```python
from build123d import *

# Parameters (mm, degrees)
F0_R     = 1
F1_DEPTH = 36
F0_R_2   = 2
F2_DEPTH = 6
F3_R     = 1
F4_R     = 1
F5_DEPTH = 25
F7_DEPTH = 100
F8_R     = 3


with BuildPart() as f1:
    # F0 (on Top) → F1 (new body)
    with BuildSketch(Plane.XY):
        with BuildLine():
            Line((-20, -12.5), (20, -12.5))
            Line((20, -12.5), (22, -12.5))
            Line((22, -12.5), (28, -12.5))
            ThreePointArc((28, -12.5), (29.414214, -11.914214), (30, -10.5))
            Line((30, -10.5), (30, 10.5))
            ThreePointArc((30, 10.5), (29.414214, 11.914214), (28, 12.5))
            Line((28, 12.5), (22, 12.5))
            Line((22, 12.5), (20, 12.5))
            Line((20, 12.5), (-20, 12.5))
            Line((-20, 12.5), (-28, 12.5))
            ThreePointArc((-28, 12.5), (-29.414214, 11.914214), (-30, 10.5))
            Line((-30, 10.5), (-30, -10.5))
            ThreePointArc((-30, -10.5), (-29.414214, -11.914214), (-28, -12.5))
            Line((-28, -12.5), (-22, -12.5))
            Line((-22, -12.5), (-20, -12.5))
        make_face()
        with Locations((-26, -6)):
            Circle(F0_R, mode=Mode.SUBTRACT)
        with Locations((26, -6)):
            Circle(F0_R, mode=Mode.SUBTRACT)
        with Locations((-26, 6)):
            Circle(F0_R, mode=Mode.SUBTRACT)
        Polygon((20.75, -10.25), (-20.75, -10.25), (-20.75, 10.25), (20.75, 10.25), (20.75, 5), (23.25, 5), (23.25, -5), (20.75, -5), align=None, mode=Mode.SUBTRACT)
        with Locations((26, 6)):
            Circle(F0_R, mode=Mode.SUBTRACT)
    extrude(amount=F1_DEPTH)

    # F0 (on Top) → F2 (join)
    with BuildSketch(Plane.XY):
        with BuildLine():
            ThreePointArc((-22, -14.5), (-21.414214, -13.085786), (-20, -12.5))
            Line((-20, -12.5), (-22, -12.5))
            Line((-22, -12.5), (-28, -12.5))
            ThreePointArc((-28, -12.5), (-29.414214, -11.914214), (-30, -10.5))
            Line((-30, -10.5), (-30, -12.5))
            Line((-30, -12.5), (-30, -18.5))
            ThreePointArc((-30, -18.5), (-29.414214, -19.914214), (-28, -20.5))
            Line((-28, -20.5), (-24, -20.5))
            ThreePointArc((-24, -20.5), (-22.585786, -19.914214), (-22, -18.5))
            Line((-22, -18.5), (-22, -14.5))
        make_face()
        with Locations((-26, -16.5)):
            Circle(F0_R_2, mode=Mode.SUBTRACT)
        with BuildLine():
            Line((22, -12.5), (20, -12.5))
            ThreePointArc((20, -12.5), (21.414214, -13.085786), (22, -14.5))
            Line((22, -14.5), (22, -18.5))
            ThreePointArc((22, -18.5), (22.585786, -19.914214), (24, -20.5))
            Line((24, -20.5), (28, -20.5))
            ThreePointArc((28, -20.5), (29.414214, -19.914214), (30, -18.5))
            Line((30, -18.5), (30, -12.5))
            Line((30, -12.5), (30, -10.5))
            ThreePointArc((30, -10.5), (29.414214, -11.914214), (28, -12.5))
            Line((28, -12.5), (22, -12.5))
        make_face()
        with Locations((26, -16.5)):
            Circle(F0_R_2, mode=Mode.SUBTRACT)
        with BuildLine():
            ThreePointArc((28, 12.5), (29.414214, 11.914214), (30, 10.5))
            Line((30, 10.5), (30, 12.5))
            Line((30, 12.5), (30, 18.5))
            ThreePointArc((30, 18.5), (29.414214, 19.914214), (28, 20.5))
            Line((28, 20.5), (24, 20.5))
            ThreePointArc((24, 20.5), (22.585786, 19.914214), (22, 18.5))
            Line((22, 18.5), (22, 14.5))
            ThreePointArc((22, 14.5), (21.414214, 13.085786), (20, 12.5))
            Line((20, 12.5), (22, 12.5))
            Line((22, 12.5), (28, 12.5))
        make_face()
        with Locations((26, 16.5)):
            Circle(F0_R_2, mode=Mode.SUBTRACT)
        with BuildLine():
            Line((-30, 12.5), (-30, 10.5))
            ThreePointArc((-30, 10.5), (-29.414214, 11.914214), (-28, 12.5))
            Line((-28, 12.5), (-20, 12.5))
            ThreePointArc((-20, 12.5), (-21.414214, 13.085786), (-22, 14.5))
            Line((-22, 14.5), (-22, 18.5))
            ThreePointArc((-22, 18.5), (-22.585786, 19.914214), (-24, 20.5))
            Line((-24, 20.5), (-28, 20.5))
            ThreePointArc((-28, 20.5), (-29.414214, 19.914214), (-30, 18.5))
            Line((-30, 18.5), (-30, 12.5))
        make_face()
        with Locations((-26, 16.5)):
            Circle(F0_R_2, mode=Mode.SUBTRACT)
        Polygon((20.75, 0), (20.75, -5), (23.25, -5), (23.25, 5), (20.75, 5), align=None)
    extrude(amount=F2_DEPTH)

    # F3
    f3_edges = [f1.edges().sort_by_distance(p)[0] for p in [
        (0, 10.25, 36),
        (-20.75, 0, 36),
        (20.75, 7.625, 36),
        (20.75, -7.625, 36),
        (0, -10.25, 36),
        (22, -5, 36),
        (23.25, 0, 36),
        (22, 5, 36),
    ]]
    fillet(f3_edges, radius=F3_R)

    # F4
    f4_edges = [f1.edges().sort_by_distance(p)[0] for p in [
        (30, 0, 36),
        (0, 12.5, 36),
        (0, -12.5, 36),
        (29.414214, -11.914214, 36),
        (29.414214, 11.914214, 36),
        (-30, 0, 36),
        (-29.414214, 11.914214, 36),
        (-29.414214, -11.914214, 36),
    ]]
    fillet(f4_edges, radius=F4_R)

    # F0 (on Top) → F5 (join)
    with BuildSketch(Plane.XY):
        with Locations((-26, 6)):
            Circle(F0_R)
        with Locations((-26, -6)):
            Circle(F0_R)
        with Locations((26, -6)):
            Circle(F0_R)
        with Locations((26, 6)):
            Circle(F0_R)
    extrude(amount=F5_DEPTH)

    # F6 (on face) → F7 (cut)
    with BuildSketch(Plane.YZ.offset(30)):
        Polygon((-9.5, 6), (9.5, 6), (9.5, 16), (0, 32.49523), (-9.5, 16), align=None)
    extrude(amount=-F7_DEPTH, mode=Mode.SUBTRACT)

    # F8
    f8_edges = [f1.edges().sort_by_distance(p)[0] for p in [
        (25.375, -9.5, 6),
        (-25.375, -9.5, 6),
        (25.375, 9.5, 6),
        (-25.375, 9.5, 6),
        (25.375, 9.5, 16),
        (-25.375, 9.5, 16),
        (25.375, -9.5, 16),
        (-25.375, -9.5, 16),
    ]]
    fillet(f8_edges, radius=F8_R)


solid = f1.part
```
Verification items for the finished model (mm, model axes). A direction names the side the tool comes from. Round coordinates to 2 decimals unless told otherwise and drop trailing zeros. Order: outer loops, then holes, each group sorted by start corner. A loop starts at its lowest first (then second) coordinate and runs counter-clockwise, first axis right, second up. Notation, with made-up numbers: (-38.75, 33) -> (-5.75, 33) arc R17 cw to (-5.75, 63) -> close; hole circle Ø4 at (38.5, -25). An arc over 180 degrees is marked (long way). Put each result on its own line as item: value. Start each with the question number.
(1) Draft check along Z on faces 1 (the face through (-25, 9.5, 12)), 2 (the face through (-26, -14, 6)), 3 (the face through (-22, 16, 3)). Enter one of: +Z half, -Z half, draft (parallel to the pull), parting line (faces both ways), or undercut.
(2) Material ranges on line 1 along Y through (x, z) = (-26, 2.1); line 2 along Y through (x, z) = (26, 33.75); line 3 along X through (y, z) = (-10, 6), recorded low to high.
(3) Section check B-B (z = 27.5). Enter the section's corners in (x, y).
(4) Section check D-D (x = -26). State how many separate pieces and enclosed holes the cut face has, then the cut area to 3 significant figures.
(5) Depth check by flat-ended pin: pin 1 Ø5 at (x, z) = (-24.5, 13) entering from +Y; pin 2 Ø6 at (x, z) = (16, 24) entering from -Y; pin 3 Ø8 at (x, y) = (-25.5, -17) entering from +Z. Enter the tip coordinate at first touch or a pass-through.
(6) Tool access check on faces 4 (the face through (29.4, -11.93, 20.3)), 5 (the face through (-20.75, -7, 21)), 6 (the face through (29.43, 11.9, 20.3)), 7 (the face through (-25, 0, 6)), 8 (the face through (26, 7, 30)). Record the directions out of +Z, -Z, +X, -X, +Y, -Y that give a thin tool (end or side, any length) a straight path to the whole face; none if there is none.
(7) Section check A-A (x = -3). Enter the section's corners in (y, z).
(8) Section check C-C (y = 3.5). Enter the section's corners in (x, z), then the cut area to 3 significant figures.
Completed:
1. face 1: undercut
1. face 2: +Z half
1. face 3: draft
2. line 1: y = -20.5 to -18.5, -14.5 to 14.5, 18.5 to 20.5
2. line 2: y = -12.5 to -7, -5 to 5, 7 to 12.5
2. line 3: x = -30 to -20.75, 20.75 to 30
3. outline: (-30, -10.5) arc R2 ccw to (-28, -12.5) -> (28, -12.5) arc R2 ccw to (30, -10.5) -> (30, -2.88) -> (23.25, -2.88) -> (23.25, -5) -> (20.75, -5) -> (20.75, -10.25) -> (-20.75, -10.25) -> (-20.75, -2.88) -> (-30, -2.88) -> close; (-30, 2.88) -> (-20.75, 2.88) -> (-20.75, 10.25) -> (20.75, 10.25) -> (20.75, 5) -> (23.25, 5) -> (23.25, 2.88) -> (30, 2.88) -> (30, 10.5) arc R2 ccw to (28, 12.5) -> (-28, 12.5) arc R2 ccw to (-30, 10.5) -> close; hole circle Ø2 at (-26, -6); hole circle Ø2 at (-26, 6); hole circle Ø2 at (26, -6); hole circle Ø2 at (26, 6)
4. separate pieces: 3
4. enclosed holes: 1
4. area: 561 mm2
5. pin 1: stops at y = 12.5
5. pin 2: stops at y = -12.5
5. pin 3: stops at z = 6
6. face 4: +Z, +X, -Y
6. face 5: +Z, -Z
6. face 6: +Z, +X, +Y
6. face 7: +X, -X
6. face 8: +Z
7. outline: (-12.5, 0) -> (-10.25, 0) -> (-10.25, 35) arc R1 ccw to (-11.25, 36) -> (-11.5, 36) arc R1 ccw to (-12.5, 35) -> close; (10.25, 0) -> (12.5, 0) -> (12.5, 35) arc R1 ccw to (11.5, 36) -> (11.25, 36) arc R1 ccw to (10.25, 35) -> close
8. outline: (-30, 0) -> (-20.75, 0) -> (-20.75, 6) -> (-30, 6) -> close; (-30, 26.42) -> (-20.75, 26.42) -> (-20.75, 35) arc R1 ccw to (-21.75, 36) -> (-29, 36) arc R1 ccw to (-30, 35) -> close; (20.75, 0) -> (30, 0) -> (30, 6) -> (20.75, 6) -> close; (23.25, 26.42) -> (30, 26.42) -> (30, 35) arc R1 ccw to (29, 36) -> (24.25, 36) arc R1 ccw to (23.25, 35) -> close
8. area: 263 mm2
